Source: CAD feature listing. Evaluate the final solid. Frame: model axes, mm. A direction names the side the tool comes from. Coordinates: 2 decimals unless noted, no trailing zeros. Loops run counter-clockwise (first coordinate to the right, second up) from the corner with the lowest first, then second, coordinate; pieces in that order, holes last. Notation, with made-up numbers: (26, 56) -> (63, 56) arc R14 ccw to (63, 73) -> close; hole circle Ø2 at (78.5, 13). An arc over 180 degrees is marked (long way). Answer as a JSON object with one key per item and string values. Group by question number.
from build123d import *

# Parameters (mm, degrees)
BOSS_EXTRUDE1_DEPTH = 100
SKETCH2_R           = 4
CUT_EXTRUDE1_DEPTH  = 200
CUT_EXTRUDE2_DEPTH  = 200
SCALE1_SCALE        = 2


with BuildPart() as part:
    # Sketch1 → Boss-Extrude1 (new, symmetric)
    with BuildSketch(Plane(origin=(0, 0, 0), x_dir=(0, 0, -1), z_dir=(1, 0, 0))):
        with BuildLine():
            Line((4.403376918, 32.272727273), (-5.596623082, 32.272727273))
            ThreePointArc((-5.596623082, 32.272727273), (-9.132156988, 30.808261179), (-10.596623082, 27.272727273))
            Line((-10.596623082, 27.272727273), (-10.596623082, -32.727272727))
            ThreePointArc((-10.596623082, -32.727272727), (-12.061089177, -36.262806633), (-15.596623082, -37.727272727))
            Line((-15.596623082, -37.727272727), (-40.596623082, -37.727272727))
            Line((-40.596623082, -37.727272727), (-40.596623082, -39.727272727))
            Line((-40.596623082, -39.727272727), (-15.596623082, -39.727272727))
            ThreePointArc((-15.596623082, -39.727272727), (-10.646875614, -37.677020196), (-8.596623082, -32.727272727))
            Line((-8.596623082, -32.727272727), (-8.596623082, 27.272727273))
            ThreePointArc((-8.596623082, 27.272727273), (-7.717943426, 29.394047616), (-5.596623082, 30.272727273))
            Line((-5.596623082, 30.272727273), (4.403376918, 30.272727273))
            Line((4.403376918, 30.272727273), (4.403376918, 32.272727273))
        make_face()
    extrude(amount=BOSS_EXTRUDE1_DEPTH, both=True)

    # Sketch2 → Cut-Extrude1 (cut)
    with BuildSketch(Plane(origin=(0, 32.272727273, 0), x_dir=(1, 0, 0), z_dir=(0, 1, 0))):
        with Locations(Location((0, -27.707416892, 0), (0, 0, 270))):
            Circle(SKETCH2_R)
        with Locations(Location((-62.576946362, -27.707416892, 0), (0, 0, 270))):
            Circle(SKETCH2_R)
        with Locations(Location((67.371990144, -27.707416892, 0), (0, 0, 270))):
            Circle(SKETCH2_R)
        with BuildLine():
            Line((-88.753028946, -40.596623082), (-100, -40.596623082))
            Line((-100, -40.596623082), (-100, -29.349652028))
            ThreePointArc((-100, -29.349652028), (-96.705838446, -37.302461529), (-88.753028946, -40.596623082))
        make_face()
        with BuildLine():
            Line((100, -40.596623082), (100, -29.349652028))
            ThreePointArc((100, -29.349652028), (96.705838446, -37.302461529), (88.753028946, -40.596623082))
            Line((88.753028946, -40.596623082), (100, -40.596623082))
        make_face()
    extrude(amount=-CUT_EXTRUDE1_DEPTH, mode=Mode.SUBTRACT)

    # Sketch3 → Cut-Extrude2 (cut)
    with BuildSketch(Plane.XY.offset(10.596623082)):
        with BuildLine():
            Line((-64.584534402, 178.454407754), (64.584534402, 178.454407754))
            Line((64.584534402, 178.454407754), (64.584534402, -16.573121652))
            ThreePointArc((64.584534402, -16.573121652), (63.120068308, -20.108655558), (59.584534402, -21.573121652))
            Line((59.584534402, -21.573121652), (-59.584534402, -21.573121652))
            ThreePointArc((-59.584534402, -21.573121652), (-63.120068308, -20.108655558), (-64.584534402, -16.573121652))
            Line((-64.584534402, -16.573121652), (-64.584534402, 178.454407754))
        make_face()
    extrude(amount=-CUT_EXTRUDE2_DEPTH, mode=Mode.SUBTRACT)


with BuildPart() as part_1:
    # Scale1: scaled about (0, 0, 0)
    add(part.part.scale(SCALE1_SCALE))


solid = part_1.part
1. Reachability of faces 1 (the face through (3, -75.455, 67)), 2 (the face through (126.317, -40.139, 19.221)), 3 (the face through (165, 60.545, 1)), 4 (the face through (193.586, -77.427, 74.429)) from +Z, -Z, +X, -X, +Y, -Y: full face, straight path, thin tool, end or side. Return the list, or none.
2. Section query B-B on x = 0. Return loops of the section in (y, z).
3. Mould query, pull axis X, two halves, no side actions, for faces 5 (the face through (-3.064, -77.427, 62.805)), 6 (the face through (-193.586, -77.427, 74.429)), 7 (the face through (-129.169, 22.7, 17.4)), 8 (the face through (3, -46, 17.193)). Classes: pulls with the +X half, pulls with the -X half, needs draft (parallel to the pull), parting line crosses it, or undercut.
4. Ray query, L1, parallel to Z at x = -15.5, y = -49; L2, parallel to X at y = 56, z = 20; L3, parallel to Y at x = 180, z = 61.5. Return the intervals inside material, ascending.
5. Pin query (flat end, axial travel): pin 1 Ø10 at (x, z) = (-160.5, -2.5) entering from -Y; pin 2 Ø1.5 at (y, z) = (-48.5, 14.5) entering from -X (3 decimals); pin 3 Ø12 at (x, y) = (12.5, -43.5) entering from -Z; pin 4 Ø4.5 at (x, z) = (-38, 18.5) entering from +Y. Return the tip coordinate at first contact, or that it passes through.
6. Section query C-C on y = 40.5. Return loops of the section in (x, z).
7. Section query D-D on x = 100.5. Return loops of the section in (y, z), then the cut area to 3 significant figures.
8. Section query A-A on z = -2. Return loops of the section in (x, y), then the cut area to 3 significant figures.
Solved:
{
 "1": {"face 1": "+Z, +X, -X, +Y", "face 2": "+Z, -Z, +Y", "face 3": "-Z, +X, -X, -Y", "face 4": "+Z, +X, +Y, -Y"},
 "2": {"outline": "(-79.45, 31.19) arc R14 ccw to (-65.45, 17.19) -> (-43.15, 17.19) -> (-43.15, 21.19) -> (-65.45, 21.19) arc R10 cw to (-75.45, 31.19) -> (-75.45, 47.41) -> (-79.45, 47.41) -> close; (-79.45, 63.41) -> (-75.45, 63.41) -> (-75.45, 81.19) -> (-79.45, 81.19) -> close"},
 "3": {"face 5": "undercut", "face 6": "pulls with the -X half", "face 7": "undercut", "face 8": "needs draft"},
 "4": {"L1": "17.19 to 21.19", "L2": "-200 to -129.17, 129.17 to 200", "L3": "-79.45 to -75.45"},
 "5": {"pin 1": "y = 60.55", "pin 2": "through", "pin 3": "z = 17.19", "pin 4": "y = -43.15"},
 "6": {"outline": "(-200, 17.19) -> (-129.17, 17.19) -> (-129.17, 21.19) -> (-200, 21.19) -> close; (129.17, 17.19) -> (200, 17.19) -> (200, 21.19) -> (129.17, 21.19) -> close"},
 "7": {"outline": "(-79.45, 31.19) arc R14 ccw to (-65.45, 17.19) -> (-43.15, 17.19) -> (-43.15, 21.19) -> (-65.45, 21.19) arc R10 cw to (-75.45, 31.19) -> (-75.45, 81.19) -> (-79.45, 81.19) -> close", "area": "365 mm^2"},
 "8": {"outline": "(-200, 60.55) -> (-129.17, 60.55) -> (-129.17, 64.55) -> (-200, 64.55) -> close; (129.17, 60.55) -> (200, 60.55) -> (200, 64.55) -> (129.17, 64.55) -> close", "area": "567 mm^2"}
}
